Design review of the part built by this model. Coordinates are the model's own, in mm. Coordinates: 2 decimals unless noted, no trailing zeros. Loops run counter-clockwise (first coordinate to the right, second up) from the corner with the lowest first, then second, coordinate; pieces in that order, holes last. Notation, with made-up numbers: M 42,40 L 75,40 A28 ccw 75,63 Z; hole C -29.75,32.5 d1. An arc over 180 degrees is marked long. Answer as a JSON object with one key per item and string values. Group by question number.
1. Insertion check: pin 1 (2 mm diameter, centred on x = 10, z = 6, fed in from -Y). The pin has a flat end and moves straight along its axis. Give the tip position at first contact, or say it passes through.
2. Consider section A-A (z = 0.25). State the section outline as (x, y) points.
3. To check wall thickness, follow probe 1 along X at (y, z) = (1.25, 0); probe 2 along X at (y, z) = (1.6, 4.25); probe 3 along Z at (x, y) = (18, 0.5). State the ranges of each line that lie inside material, in increasing order.
4. Consider section D-D (z = -8.75). State the section outline as (x, y) points.
5. Consider section B-B (y = 0.4). State the section outline as (x, z) points.
6. Consider section C-C (x = -33). State the section outline as (y, z) points, then the cut area to 3 significant figures.
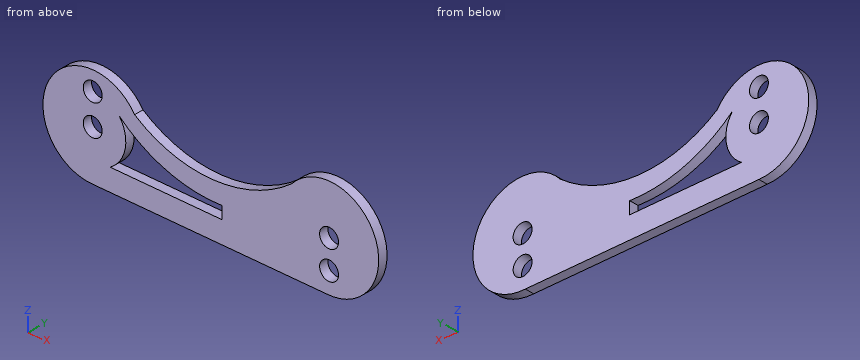
from build123d import *

# Parameters (mm, degrees)
SKETCH1_R           = 2
BOSS_EXTRUDE5_DEPTH = 2


with BuildPart() as part:
    # Sketch1 → Boss-Extrude5 (new body)
    with BuildSketch(Plane(origin=(0, 0, 0), x_dir=(1, 0, 0), z_dir=(0, 1, 0))):
        with BuildLine():
            Line((-33.661525998, 9.558347037), (15.746838945, 10.493683155))
            ThreePointArc((15.746838945, 10.493683155), (25.998283023, -4.08303674), (8.397040734, -6.870354169))
            ThreePointArc((8.397040734, -6.870354169), (-8.169868029, -1.163623151), (-24.804581512, -6.669579217))
            ThreePointArc((-24.804581512, -6.669579217), (-42.905321973, -6.017722997), (-33.661525998, 9.558347037))
        make_face()
        with Locations(Location((-33.661525998, -0.972605925, 0), (0, 0, 270))):
            Circle(SKETCH1_R, mode=Mode.SUBTRACT)
        with Locations(Location((-33.661525998, -7.472605925, 0), (0, 0, 270))):
            Circle(SKETCH1_R, mode=Mode.SUBTRACT)
        with Locations(Location((16.328821379, 0.009824302, 0), (0, 0, 270))):
            Circle(SKETCH1_R, mode=Mode.SUBTRACT)
        with Locations(Location((16.328821379, 6.009824302, 0), (0, 0, 270))):
            Circle(SKETCH1_R, mode=Mode.SUBTRACT)
        with BuildLine():
            Line((-29.996106609, 4.99100881), (-6.337353933, 5.438886126))
            Line((-6.337353933, 5.438886126), (-6.337353933, 2.841108528))
            ThreePointArc((-6.337353933, 2.841108528), (-17.995175719, 0.977836677), (-28.067473468, -5.180524211))
            ThreePointArc((-28.067473468, -5.180524211), (-26.784064544, 0.331435467), (-29.996106609, 4.99100881))
        make_face(mode=Mode.SUBTRACT)
    extrude(amount=BOSS_EXTRUDE5_DEPTH)


solid = part.part
Findings below:
{
 "1": {"pin 1": "stops at y = 0"},
 "2": {"outline": "M -44.17,0 L -35.53,0 L -35.53,2 L -44.17,2 Z; M -31.8,0 L -26.7,0 L -26.7,2 L -31.8,2 Z; M -20.86,0 L 14.35,0 L 14.35,2 L -20.86,2 Z; M 18.31,0 L 26.83,0 L 26.83,2 L 18.31,2 Z"},
 "3": {"probe 1": "x = -44.15 to -35.41, -31.91 to -26.73, -20.34 to 14.33, 18.33 to 26.83", "probe 2": "x = -43.67 to -27.48, -27.01 to -20.97, 4.29 to 25.93", "probe 3": "z = -10.38 to -7.11, -4.91 to -1.11, 1.09 to 10.36"},
 "4": {"outline": "M -37.71,0 L 22.15,0 L 22.15,2 L -37.71,2 Z"},
 "5": {"outline": "M -33.66,-9.56 L 15.75,-10.49 A10.5 ccw long 8.4,6.87 A27.38 cw -24.8,6.67 A10.53 ccw long Z; hole C -33.66,0.97 d4; hole C -33.66,7.47 d4; hole M -30,-4.99 L -6.34,-5.44 L -6.34,-2.84 A30.44 cw -28.07,5.18 A7 cw Z; hole C 16.33,-6.01 d4; hole C 16.33,-0.01 d4"},
 "6": {"outline": "M 0,-9.57 L 2,-9.57 L 2,-0.91 L 0,-0.91 Z; M 0,2.86 L 2,2.86 L 2,5.59 L 0,5.59 Z; M 0,9.36 L 2,9.36 L 2,11.48 L 0,11.48 Z", "area": "27.0 mm^2"}
}
